```python
from build123d import *

# Parameters (mm, degrees)
SKETCH_1_W             = 50
SKETCH_1_H             = 20
SKETCH_1_W_2           = 48
SKETCH_1_H_2           = 18
EXTRUDE_1_DEPTH        = 150
SKETCH_2_R             = 1.525
CUT_EXTRUDE_1_DEPTH    = 10
PATTERN_LINEAR_1_COUNT = 15
PATTERN_LINEAR_1_PITCH = 20
SKETCH_3_R             = 1.525
CUT_EXTRUDE_2_DEPTH    = 100
SKETCH_4_R             = 1.525
CUT_EXTRUDE_3_DEPTH    = 100
SKETCH_5_R             = 2.025
CUT_EXTRUDE_4_DEPTH    = 39
SKETCH_7_R             = 5.5
CUT_EXTRUDE_6_DEPTH    = 10
CUT_EXTRUDE_7_DEPTH    = 10
PATTERN_LINEAR_2_COUNT = 4
PATTERN_LINEAR_2_PITCH = 60
SKETCH_9_R             = 5.5
CUT_EXTRUDE_8_DEPTH    = 10
PATTERN_LINEAR_3_COUNT = 6
PATTERN_LINEAR_3_PITCH = 30
SKETCH_10_R            = 2.025
CUT_EXTRUDE_9_DEPTH    = 10
SKETCH_11_R            = 2.025
CUT_EXTRUDE_10_DEPTH   = 8


with BuildPart() as part:
    # 草图1 → 凸台-拉伸1 (new body, symmetric)
    with BuildSketch(Plane.XY):
        Rectangle(SKETCH_1_W, SKETCH_1_H)
        Rectangle(SKETCH_1_W_2, SKETCH_1_H_2, mode=Mode.SUBTRACT)
    extrude(amount=EXTRUDE_1_DEPTH, both=True)

    # 草图2 → 切除-拉伸1 (cut)
    with BuildSketch(Plane(origin=(0, 10, 0), x_dir=(1, 0, 0), z_dir=(0, 1, 0))):
        with Locations((-12, -140)):
            Circle(SKETCH_2_R)
        with Locations((12, -140)):
            Circle(SKETCH_2_R)
    cut_extrude_1 = extrude(amount=-CUT_EXTRUDE_1_DEPTH, mode=Mode.SUBTRACT)

    # 阵列(线性)1: 切除-拉伸1 ×15
    with Locations(*[(0, 0, -i * PATTERN_LINEAR_1_PITCH) for i in range(1, PATTERN_LINEAR_1_COUNT)]):
        add(cut_extrude_1, mode=Mode.SUBTRACT)

    # 草图3 → 切除-拉伸2 (cut)
    with BuildSketch(Plane(origin=(25, 0, 0), x_dir=(0, 0, -1), z_dir=(1, 0, 0))):
        with Locations((50, 0)):
            Circle(SKETCH_3_R)
        with Locations((20, 0)):
            Circle(SKETCH_3_R)
        with Locations((-10, 0)):
            Circle(SKETCH_3_R)
        with Locations((-40, 0)):
            Circle(SKETCH_3_R)
        with Locations((-70, 0)):
            Circle(SKETCH_3_R)
        with Locations((-100, 0)):
            Circle(SKETCH_3_R)
        with Locations((-130, 0)):
            Circle(SKETCH_3_R)
    extrude(amount=-CUT_EXTRUDE_2_DEPTH, mode=Mode.SUBTRACT)

    # 草图4 → 切除-拉伸3 (cut)
    with BuildSketch(Plane.XZ.offset(10)):
        with Locations((-19, 144)):
            Circle(SKETCH_4_R)
        with Locations((1, 144)):
            Circle(SKETCH_4_R)
    extrude(amount=-CUT_EXTRUDE_3_DEPTH, mode=Mode.SUBTRACT)

    # 草图5 → 切除-拉伸4 (cut)
    with BuildSketch(Plane.XZ.offset(10)):
        with Locations((19, 120)):
            Circle(SKETCH_5_R)
        with Locations((-19, 120)):
            Circle(SKETCH_5_R)
    extrude(amount=-CUT_EXTRUDE_4_DEPTH, mode=Mode.SUBTRACT)

    # 草图7 → 切除-拉伸6 (cut)
    with BuildSketch(Plane(origin=(0, -9, 0), x_dir=(1, 0, 0), z_dir=(0, 1, 0))):
        with Locations((-12, -100)):
            Circle(SKETCH_7_R)
        with Locations((12, -100)):
            Circle(SKETCH_7_R)
    extrude(amount=-CUT_EXTRUDE_6_DEPTH, mode=Mode.SUBTRACT)

    # 草图6 → 切除-拉伸7 (cut)
    with BuildSketch(Plane(origin=(0, -9, 0), x_dir=(1, 0, 0), z_dir=(0, 1, 0))):
        with BuildLine():
            Line((-6.5, 100), (-6.5, 80))
            ThreePointArc((-6.5, 80), (-12, 74.5), (-17.5, 80))
            Line((-17.5, 80), (-17.5, 100))
            ThreePointArc((-17.5, 100), (-12, 105.5), (-6.5, 100))
        make_face()
        with BuildLine():
            Line((6.5, 100), (6.5, 80))
            ThreePointArc((6.5, 80), (12, 74.5), (17.5, 80))
            Line((17.5, 80), (17.5, 100))
            ThreePointArc((17.5, 100), (12, 105.5), (6.5, 100))
        make_face()
    cut_extrude_7 = extrude(amount=-CUT_EXTRUDE_7_DEPTH, mode=Mode.SUBTRACT)

    # 阵列(线性)2: 切除-拉伸7 ×4
    with Locations(*[(0, 0, i * PATTERN_LINEAR_2_PITCH) for i in range(1, PATTERN_LINEAR_2_COUNT)]):
        add(cut_extrude_7, mode=Mode.SUBTRACT)

    # 草图9 → 切除-拉伸8 (cut)
    with BuildSketch(Plane.ZY.offset(25)):
        with Locations((-50, 0)):
            Circle(SKETCH_9_R)
    cut_extrude_8 = extrude(amount=-CUT_EXTRUDE_8_DEPTH, mode=Mode.SUBTRACT)

    # 阵列(线性)3: 切除-拉伸8 ×6
    with Locations(*[(0, 0, i * PATTERN_LINEAR_3_PITCH) for i in range(1, PATTERN_LINEAR_3_COUNT)]):
        add(cut_extrude_8, mode=Mode.SUBTRACT)

    # 草图10 → 切除-拉伸9 (cut)
    with BuildSketch(Plane.XZ.offset(10)):
        with Locations((19, -140)):
            Circle(SKETCH_10_R)
        with Locations((-19, -140)):
            Circle(SKETCH_10_R)
    extrude(amount=-CUT_EXTRUDE_9_DEPTH, mode=Mode.SUBTRACT)

    # 草图11 → 切除-拉伸10 (cut)
    with BuildSketch(Plane.XZ.offset(10)):
        with Locations((-19, -122)):
            Circle(SKETCH_11_R)
        with Locations((19, -122)):
            Circle(SKETCH_11_R)
    extrude(amount=-CUT_EXTRUDE_10_DEPTH, mode=Mode.SUBTRACT)


solid = part.part
```
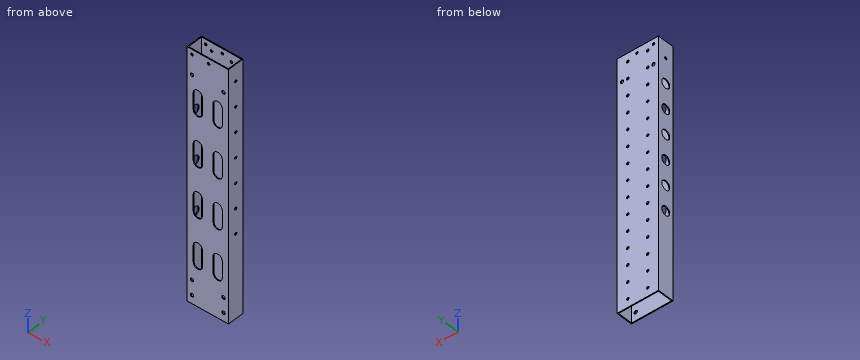
Source: CAD feature listing. Evaluate the final solid. Frame: model axes, mm. Coordinates: 2 decimals unless noted, no trailing zeros. Order: outer loops, then holes, each group sorted by start corner. A loop starts at its lowest first (then second) coordinate and runs counter-clockwise, first axis right, second up. Notation, with made-up numbers: M 77.25,46.5 L 91.25,46.5 A33 cw 91.25,76.5 Z; hole C 73,-1 d11. An arc over 180 degrees is marked long. Write each question's results on one line, items separated by ' | '. Start each with the question number.
1) Line query: line 1 (X direction, y = 9.25, z = -100) (3 decimals); line 2 (Y direction, x = 9, z = -14.5); line 3 (X direction, y = 3.5, z = 17). Output: solid intervals per line, ascending. Write a range as from..to.
2) Section query A-A (z = 90.5). Return the cut outline in (x, y).
3) Contact query for flat-ended pins moving along their axis: pin 1 Ø1.8 at (x, z) = (12, 120) entering from +Y; pin 2 Ø3.5 at (x, z) = (-19, 144) entering from -Y; pin 3 Ø1.5 at (x, z) = (11, -100.5) entering from -Y; pin 4 Ø4 at (y, z) = (0, -50) entering from -X. Output: stop coordinate, or through.
Answers:
1) line 1: x = -25..-13.525, -10.475..10.475, 13.525..25 | line 2: y = -10..-9, 9..10 | line 3: x = -25..-24, 24..25
2) outline: M -25,-10 L -17.5,-10 L -17.5,-9 L -24,-9 L -24,9 L 24,9 L 24,-9 L 17.5,-9 L 17.5,-10 L 25,-10 L 25,10 L -25,10 Z; M -6.5,-10 L 6.5,-10 L 6.5,-9 L -6.5,-9 Z
3) pin 1: stops at y = -9 | pin 2: stops at y = -10 | pin 3: stops at y = 9 | pin 4: stops at x = 24
